Can you work these out from the drawing? Everything is in mm from the part's minimum corner. A direction names the side the tool comes from. Coordinates: 2 decimals unless noted, no trailing zeros. Loops run counter-clockwise (first coordinate to the right, second up) from the corner with the lowest first, then second, coordinate; pieces in that order, holes last.
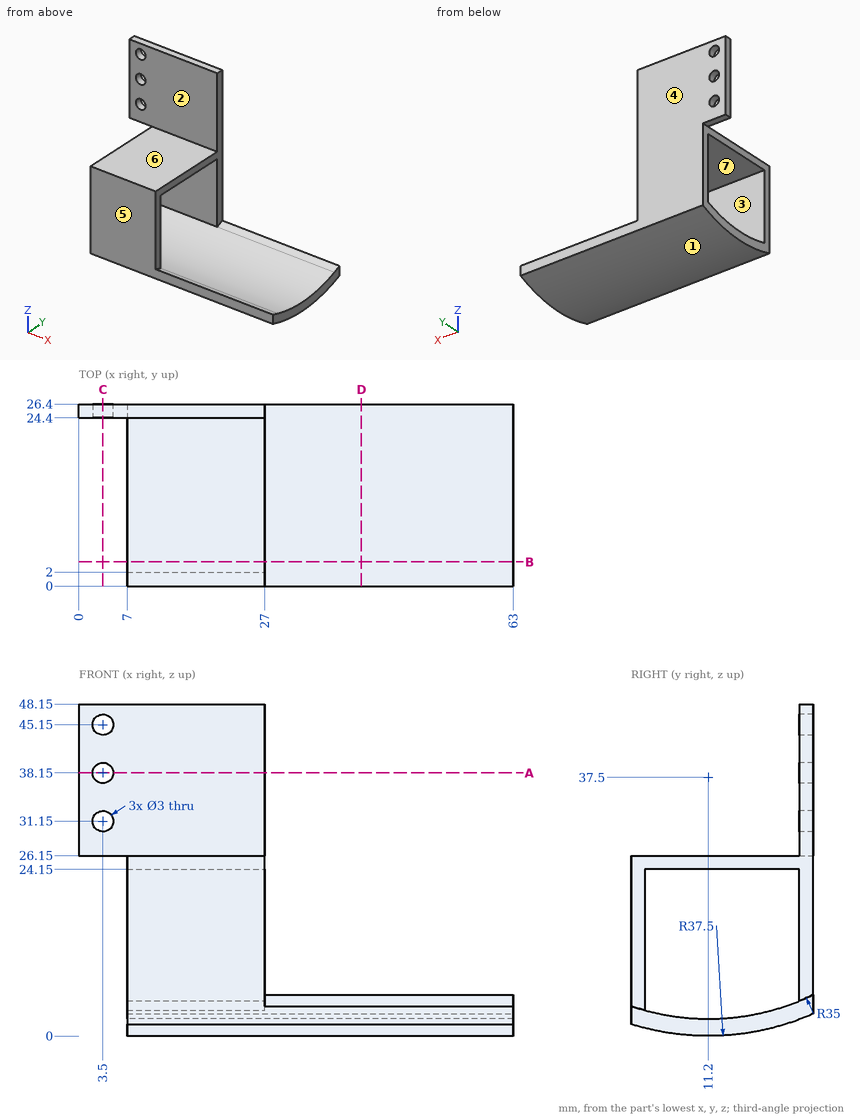
1. I want a section at C-C (x = 3.5). Please give me the cut outline in (y, z).
2. For pin 1 (6 mm diameter, centred on x = 17.5, y = 13.5, fed in from -Z); pin 2 (10 mm diameter, centred on x = 26, y = 3, fed in from +Z); pin 3 (24 mm diameter, centred on x = 16, z = 42, fed in from -Y), each with a flat end and sliding along its axis, tell me the tip position at first contact or that it passes through.
3. We'd pull the mould along Y, two halves only. Please class the marked faces 1, 2, 3 and 4: +Y half, -Y half, draft (parallel to the pull), parting line (faces both ways), or undercut.
4. I want a section at D-D (x = 41). Please give me the cut outline in (y, z), then the cut area to 3 significant figures.
5. I need wall thicknesses on line 1 along Z through (x, y) = (3.5, 25.6); line 2 along Y through (x, z) = (24, 22); line 3 along X through (y, z) = (24.5, 19.5). Which ranges of each line are inside material? Lowest first, please.
6. On a 3-axis mill with a long thin cutter (end or side, diameter ignored), from which of +Z, -Z, +X, -X, +Y, -Y can I reach the whole of each face in a straight line? I mean the marked faces 5, 6 and 7. Say none if no direction works.
7. I want a section at A-A (z = 38.15). Please give me the cut outline in (x, y).
8. I want a section at B-B (y = 3.5). Please give me the cut outline in (x, z), then the cut area to 3 significant figures.
Response values:
1. outline: (24.4, 26.15) - (26.4, 26.15) - (26.4, 29.65) - (24.4, 29.65) - close; (24.4, 32.65) - (26.4, 32.65) - (26.4, 36.65) - (24.4, 36.65) - close; (24.4, 39.65) - (26.4, 39.65) - (26.4, 43.65) - (24.4, 43.65) - close; (24.4, 46.65) - (26.4, 46.65) - (26.4, 48.15) - (24.4, 48.15) - close
2. pin 1: stops at z = 0
2. pin 2: stops at z = 26.15
2. pin 3: stops at y = 24.4
3. face 1: parting line
3. face 2: -Y half
3. face 3: undercut
3. face 4: +Y half
4. outline: (0, 1.71) arc R37.5 ccw to (26.4, 3.22) - (26.4, 5.97) arc R35 cw to (0, 4.34) - close
4. area: 67.7 mm2
5. line 1: z = 26.15 to 29.65, 32.65 to 36.65, 39.65 to 43.65, 46.65 to 48.15
5. line 2: y = 0 to 2, 24.4 to 26.4
5. line 3: x = 7 to 27
6. face 5: +Z, -Z, +X, -X, -Y
6. face 6: +Z, +X, -X, -Y
6. face 7: +X, -X
7. outline: (0, 24.4) - (2, 24.4) - (2, 26.4) - (0, 26.4) - close; (5, 24.4) - (27, 24.4) - (27, 26.4) - (5, 26.4) - close
8. outline: (7, 0.8) - (63, 0.8) - (63, 3.36) - (7, 3.36) - close; (7, 24.15) - (27, 24.15) - (27, 26.15) - (7, 26.15) - close
8. area: 183 mm2
